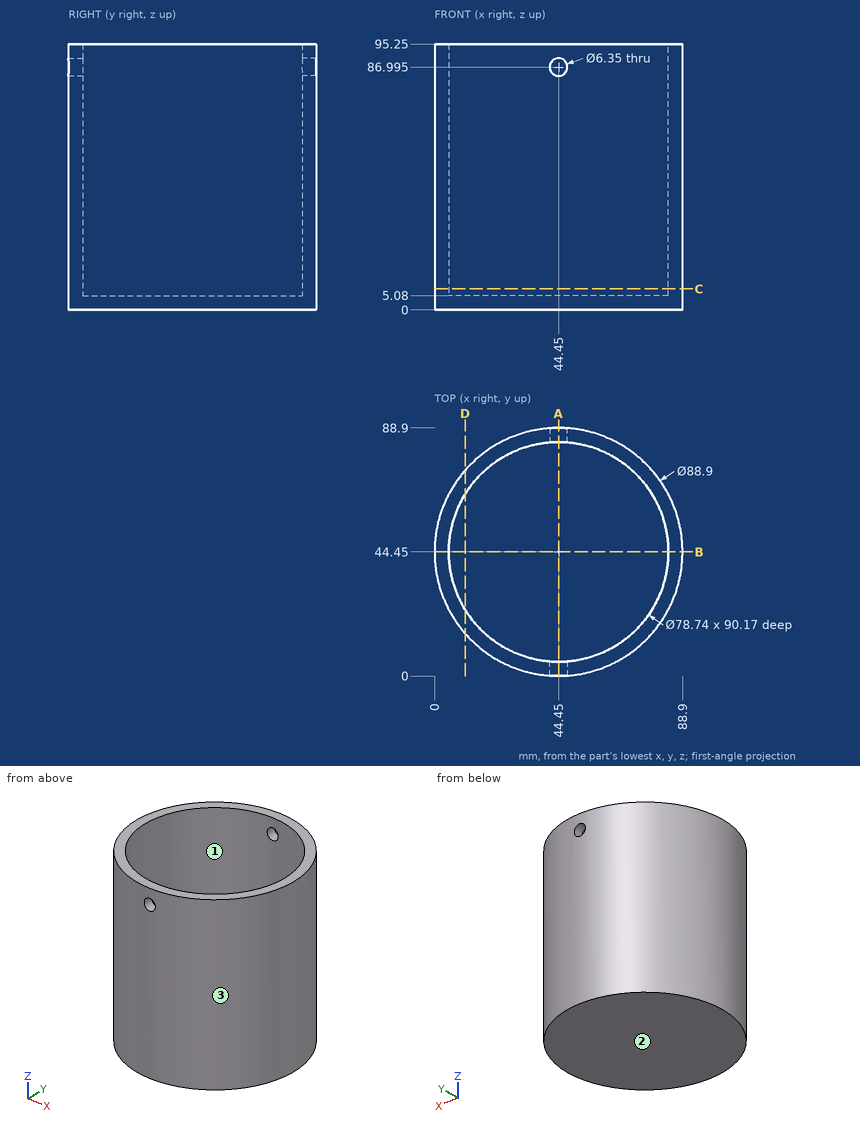
Study the drawing (mm; zero at the part's minimum x, y, z) and answer. Coordinates: 2 decimals unless noted, no trailing zeros. Loops run counter-clockwise (first coordinate to the right, second up) from the corner with the lowest first, then second, coordinate; pieces in that order, holes last. Notation, with made-up numbers: M -38.5,82.5 L 7.5,82.5 A12 ccw 7.5,92.5 Z; hole C 61,-32 d11. An arc over 180 degrees is marked long. Answer as a JSON object with one key per item and string values. Group by question number.
Item 1: Consider L1, parallel to Z at x = 44.45, y = 2.1; L2, parallel to Z at x = 44, y = 86; L3, parallel to Y at x = 44.45, z = 52. Determine where each line is inside the solid, lowest interval first.
Item 2: Section B-B (y = 44.45) is taken. Write down the section's boundary in (x, z), and give its area (3 significant figures).
Item 3: Determine the mould class of the marked faces 1, 2 and 3 for opening direction X: +X half, -X half, draft (parallel to the pull), parting line (faces both ways), or undercut.
Item 4: Each of these flat-tipped pins is pushed along its axis until it touches: P1, Ø6, axis at x = 38.5, z = 76.5, coming from the +Y side; P2, Ø4, axis at y = 29, z = 25.5, coming from the -X side; P3, Ø1, axis at y = 13, z = 75.5, coming from the -X side; P4, Ø5, axis at x = 44.45, z = 86.995, coming from the +Y side. Where does it stop, or does it pass through?
Item 5: Section A-A (x = 44.45) is taken. Write down the section's boundary in (y, z), and give its area (3 significant figures).
Item 6: Section D-D (x = 11) is taken. Write down the section's boundary in (y, z), and give its area (3 significant figures).
Item 7: Section C-C (z = 7.5) is taken. Write down the section's boundary in (x, y).
Solved:
{
 "1": {"L1": "z = 0 to 83.82, 90.17 to 95.25", "L2": "z = 0 to 83.85, 90.14 to 95.25", "L3": "y = 0 to 5.08, 83.82 to 88.9"},
 "2": {"outline": "M 0,0 L 88.9,0 L 88.9,95.25 L 83.82,95.25 L 83.82,5.08 L 5.08,5.08 L 5.08,95.25 L 0,95.25 Z", "area": "1,370 mm2"},
 "3": {"face 1": "undercut", "face 2": "draft", "face 3": "parting line"},
 "4": {"P1": "stops at y = 88.8", "P2": "stops at x = 2.08", "P3": "stops at x = 12.55", "P4": "passes through"},
 "5": {"outline": "M 0,0 L 88.9,0 L 88.9,83.82 L 83.82,83.82 L 83.82,5.08 L 5.08,5.08 L 5.08,83.82 L 0,83.82 Z; M 0,90.17 L 5.08,90.17 L 5.08,95.25 L 0,95.25 Z; M 83.82,90.17 L 88.9,90.17 L 88.9,95.25 L 83.82,95.25 Z", "area": "1,300 mm2"},
 "6": {"outline": "M 15.18,0 L 73.72,0 L 73.72,95.25 L 65.21,95.25 L 65.21,5.08 L 23.69,5.08 L 23.69,95.25 L 15.18,95.25 Z", "area": "1,830 mm2"},
 "7": {"outline": "C 44.45,44.45 d88.9; hole C 44.45,44.45 d78.74"}
}
